Input: part model. Units: mm. Frame: model coordinates. A direction names the side the tool comes from. Give positions to 0.01 mm unless a question says otherwise; leave off trailing zeros. Write each loop counter-clockwise with the first axis right and the second up, starting at its lowest first coordinate (ties: lowest second). Pieces come first, ordered by that corner, then holes. Notation, with made-up numbers: (88.25, 29.25) - (111.25, 29.25) arc R26 ccw to (111.25, 68.25) - close; hole circle Ø3 at (80.25, 78). An arc over 180 degrees is marked (long way). Answer as CSV lines item,"result".
```python
from build123d import *

# Parameters (mm, degrees)
BOSS_EXTRUDE1_DEPTH  = 14
SKETCH20_W           = 41
SKETCH20_H           = 14
BOSS_EXTRUDE10_DEPTH = 5
SKETCH21_R           = 2.65
CUT_EXTRUDE13_DEPTH  = 5
SKETCH22_W           = 5
SKETCH22_H           = 4
CUT_EXTRUDE14_DEPTH  = 59.966091951
SKETCH23_R           = 2.65
BOSS_EXTRUDE11_DEPTH = 5
SKETCH24_W           = 25
SKETCH24_H           = 7
CUT_EXTRUDE15_DEPTH  = 3
CUT_EXTRUDE16_REACH  = 65.285
SKETCH25_W           = 12
SKETCH25_H           = 7


with BuildPart() as part:
    # Sketch1 → Boss-Extrude1 (new body)
    with BuildSketch(Plane(origin=(0, 0, 0), x_dir=(1, 0, 0), z_dir=(0, 1, 0))):
        Polygon((6.589095597, 0), (10, 0), (10, 4), (40, 4), (40, 9), (11.589095597, 9), (0, 9), (0, 0), align=None)
    extrude(amount=BOSS_EXTRUDE1_DEPTH)

    # Sketch20 → Boss-Extrude10 (add)
    with BuildSketch(Plane.ZY):
        with Locations((20.5, 7)):
            Rectangle(SKETCH20_W, SKETCH20_H)
    extrude(amount=-BOSS_EXTRUDE10_DEPTH)

    # Sketch21 → Cut-Extrude13 (cut)
    with BuildSketch(Plane.ZY):
        with Locations((-4.35, 7)):
            Circle(SKETCH21_R)
        with Locations((3.65, 7)):
            Circle(SKETCH21_R)
        with Locations((11.65, 7)):
            Circle(SKETCH21_R)
        with Locations((19.65, 7)):
            Circle(SKETCH21_R)
        with Locations((27.65, 7)):
            Circle(SKETCH21_R)
        with Locations((35.65, 7)):
            Circle(SKETCH21_R)
    extrude(amount=-CUT_EXTRUDE13_DEPTH, mode=Mode.SUBTRACT)

    # Sketch22 → Cut-Extrude14 (cut, through all)
    with BuildSketch(Plane(origin=(0, 14, 0), x_dir=(1, 0, 0), z_dir=(0, 1, 0))):
        with Locations((7.5, 2)):
            Rectangle(SKETCH22_W, SKETCH22_H)
    extrude(amount=-CUT_EXTRUDE14_DEPTH, mode=Mode.SUBTRACT)

    # Sketch23 → Boss-Extrude11 (add)
    with BuildSketch(Plane.ZY):
        with Locations((-4.35, 7)):
            Circle(SKETCH23_R)
    extrude(amount=-BOSS_EXTRUDE11_DEPTH)

    # Sketch24 → Cut-Extrude15 (cut)
    with BuildSketch(Plane(origin=(0, 0, -9), x_dir=(-1, 0, 0), z_dir=(0, 0, -1))):
        with Locations((-24.5, 7)):
            Rectangle(SKETCH24_W, SKETCH24_H)
    extrude(amount=-CUT_EXTRUDE15_DEPTH, mode=Mode.SUBTRACT)

    # Sketch25 → Cut-Extrude16 (cut, up to next)
    with BuildSketch(Plane(origin=(0, 0, -6), x_dir=(-1, 0, 0), z_dir=(0, 0, -1)), mode=Mode.PRIVATE) as cut_extrude16_sk1:
        with Locations((-24.5, 7)):
            Rectangle(SKETCH25_W, SKETCH25_H)
    cut_extrude16_tool1 = extrude(cut_extrude16_sk1.sketch, amount=-CUT_EXTRUDE16_REACH, mode=Mode.PRIVATE) & part.part
    add(cut_extrude16_tool1.solids().sort_by_distance((24.5, 7, -6))[0], mode=Mode.SUBTRACT)


solid = part.part
```
Item 1: Mould query, pull axis Z, two halves, no side actions, for faces 4 (the face through (5, 4, 18)), 5 (the face through (2, 7, 33)), 6 (the face through (18, 7, -4)). Classes: +Z half, -Z half, draft (parallel to the pull), parting line (faces both ways), or undercut.
The answers:
face 4,"draft"
face 5,"undercut"
face 6,"+Z half"
Item 2: Cut plane A-A on z = 35.65. Return the cut outline in (x, y).
The answers:
outline,"(0, 0) - (5, 0) - (5, 4.35) - (0, 4.35) - close; (0, 9.65) - (5, 9.65) - (5, 14) - (0, 14) - close"
Item 3: Ray query, line 1 (Y direction, x = 1, z = 19.65); line 2 (X direction, y = 7.25, z = 32); line 3 (Z direction, x = 32, y = 6). Return the intervals inside material, ascending. Write a range as from..to.
The answers:
line 1,"0..4.35, 9.65..14"
line 2,"0..5"
line 3,"-6..-4"
Item 4: Contact query for flat-ended pins moving along their axis: pin 1 (3 mm diameter, centred on x = 15.5, y = 6, fed in from -Z); pin 2 (7 mm diameter, centred on y = 7, z = 27.65, fed in from +X); pin 3 (2.5 mm diameter, centred on y = 7.5, z = -8, fed in from -X). Output: stop coordinate, or through.
The answers:
pin 1,"z = -6"
pin 2,"x = 5"
pin 3,"x = 0"
Item 5: Cut plane C-C on y = 7. Count the separate pieces of the cut face and the enclosed holes in it, plus the area to 4 significant figures.
The answers:
separate pieces,"7"
enclosed holes,"0"
area,"193.5 mm²"
Item 6: Cut plane B-B on x = 32. Return the cut outline in (y, z), plus the area to 3 significant figures.
The answers:
outline,"(0, -9) - (3.5, -9) - (3.5, -6) - (10.5, -6) - (10.5, -9) - (14, -9) - (14, -4) - (0, -4) - close"
area,"49.0 mm²"
Item 7: Cut plane D-D on z = -1. Return the cut outline in (x, y), plus the area to 3 significant figures.
The answers:
outline,"(0, 0) - (5, 0) - (5, 14) - (0, 14) - close"
area,"70.0 mm²"
Item 8: Reachability of faces 1 (the face through (4, 0, 5)), 2 (the face through (25, 10.5, -7)), 3 (the face through (30.5, 7, -5)) from +Z, -Z, +X, -X, +Y, -Y: full face, straight path, thin tool, end or side. Return the list, or none.
The answers:
face 1,"+Z, -Z, +X, -X, -Y"
face 2,"-Z"
face 3,"+Z, -Z"
